Can you work these out from the drawing? Everything is in mm from the part's minimum corner. A direction names the side the tool comes from. Coordinates: 2 decimals unless noted, no trailing zeros. Order: outer loops, then holes, each group sorted by start corner. A loop starts at its lowest first (then second) coordinate and runs counter-clockwise, first axis right, second up. Notation, with made-up numbers: (-18.5, 27.5) -> (-3.5, 27.5) arc R15 ccw to (-3.5, 39.5) -> close; hole circle Ø10 at (18.25, 60.25). An arc over 180 degrees is marked (long way). Return JSON: item names as keys, results as strings. Group by question number.
1) If we section it at C-C, the plane y = 28: Please give me the cut outline in (x, z), then the cut area to 3 significant figures.
2) If we section it at A-A, the plane y = 10.75: Please give me the cut outline in (x, z).
3) For pin 1 (4 mm diameter, centred on x = 24, z = 4, fed in from +Y); pin 2 (7 mm diameter, centred on x = 10.75, y = 10.75, fed in from +Z), each with a flat end and sliding along its axis, tell me the tip position at first contact or that it passes through.
4) For the marked faces 5 and 6, which set-ups out of +Z, -Z, +X, -X, +Y, -Y let a thin tool reach every point of the face, with its end or its side?
5) Thinking about a two-plate mould opening in Y: for the marked faces 1, 2, 3 and 4, which applies, +Y half, -Y half, draft (parallel to the pull), parting line (faces both ways), or undercut?
6) If we section it at D-D, the plane z = 0.5: Please give me the cut outline in (x, y), then the cut area to 3 significant figures.
7) If we section it at B-B, the plane x = 10.75: Please give me the cut outline in (y, z), then the cut area to 3 significant figures.
8) If I drill on probe 1 along Z at (x, y) = (41, 23.5); probe 2 along Y at (x, z) = (38.25, 3.75); probe 3 along X at (y, z) = (11, 9), over which ranges is the centre line in solid material (lowest first)? Write a range as from..to.
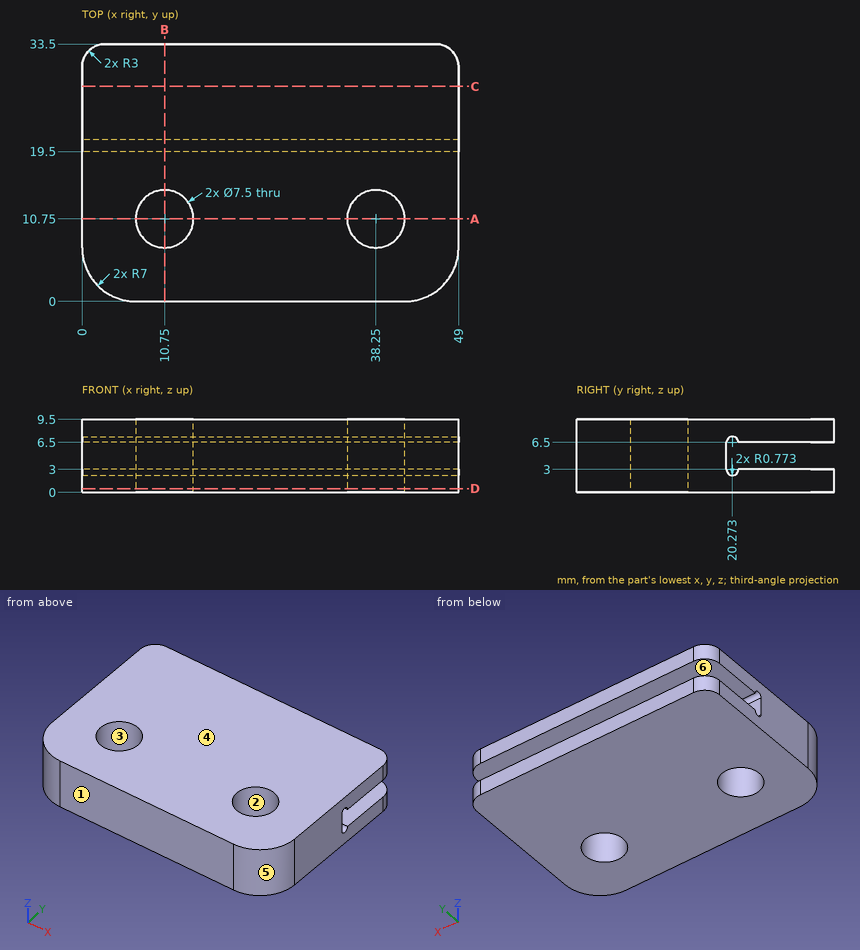
Result sheet:
{
 "1": {"outline": "(0, 0) -> (49, 0) -> (49, 3) -> (0, 3) -> close; (0, 6.5) -> (49, 6.5) -> (49, 9.5) -> (0, 9.5) -> close", "area": "294 mm2"},
 "2": {"outline": "(0, 0) -> (7, 0) -> (7, 9.5) -> (0, 9.5) -> close; (14.5, 0) -> (34.5, 0) -> (34.5, 9.5) -> (14.5, 9.5) -> close; (42, 0) -> (49, 0) -> (49, 9.5) -> (42, 9.5) -> close"},
 "3": {"pin 1": "stops at y = 33.5", "pin 2": "passes through"},
 "4": {"face 5": "+Z, -Z, +X, -Y", "face 6": "+X, -X, +Y"},
 "5": {"face 1": "-Y half", "face 2": "undercut", "face 3": "undercut", "face 4": "draft"},
 "6": {"outline": "(0, 7) arc R7 ccw to (7, 0) -> (42, 0) arc R7 ccw to (49, 7) -> (49, 30.5) arc R3 ccw to (46, 33.5) -> (3, 33.5) arc R3 ccw to (0, 30.5) -> close; hole circle Ø7.5 at (10.75, 10.75); hole circle Ø7.5 at (38.25, 10.75)", "area": "1,530 mm2"},
 "7": {"outline": "(0, 0) -> (7, 0) -> (7, 9.5) -> (0, 9.5) -> close; (14.5, 0) -> (33.5, 0) -> (33.5, 3) -> (21.05, 3) arc R0.77 cw to (19.5, 3) -> (19.5, 6.5) arc R0.77 cw to (21.05, 6.5) -> (33.5, 6.5) -> (33.5, 9.5) -> (14.5, 9.5) -> close", "area": "196 mm2"},
 "8": {"probe 1": "z = 0..3, 6.5..9.5", "probe 2": "y = 0..7, 14.5..19.5", "probe 3": "x = 0..7.01, 14.49..34.51, 41.99..49"}
}
